The figure shows three views and two pictorial views of one solid part (mm, origin at its lowest corner). Answer the questions. A direction names the side the tool comes from. Coordinates: 2 decimals unless noted, no trailing zeros. Loops run counter-clockwise (first coordinate to the right, second up) from the corner with the lowest first, then second, coordinate; pieces in that order, holes last. Notation, with made-up numbers: M 29.25,52 L 86.25,52 A26 cw 86.25,75 Z; hole C 84.25,27 d6. An arc over 180 degrees is marked long. Answer as a JSON object with one key per item and string values. Group by question number.
1. For the marked faces 5, 6 and 7, determine the directions among +Z, -Z, +X, -X, +Y, -Y from which every point of the face is accessible in a straight line to the end or side of a thin tool.
2. Determine the mould class of the marked faces 1, 2, 3 and 4 for opening direction Z: released by +Z, released by -Z, zero draft, split by the parting line, or undercut.
3. A cutting plane is placed at A-A on x = 70. Give the vertices of the cut face in (y, z), and give its area (3 significant figures).
4. Straight lines are drawn through the part: L1, parallel to X at y = 8, z = 30; L2, parallel to X at y = 11.5, z = 38.5; L3, parallel to Z at x = 108, y = 5. For each, find the intervals that lie inside material, in ascending order.
5. Given pin 1 (6 mm diameter, centred on x = 29, y = 12, fed in from +Z); pin 2 (10 mm diameter, centred on y = 6, z = 24, fed in from +X); pin 3 (4 mm diameter, centred on y = 4, z = 34.5, fed in from -X); pin 4 (8 mm diameter, centred on x = 103, z = 52.5, fed in from -Y), each flat-ended and moving along its own axis, determine where each tip first touches the part or whether it passes through.
6. A cutting plane is placed at B-B on y = 11. Give the vertices of the cut face in (x, z), and give its area (3 significant figures).
7. A cutting plane is placed at C-C on z = 30. Give the vertices of the cut face in (x, y).
8. A cutting plane is placed at D-D on x = 35.5. Give the vertices of the cut face in (y, z).
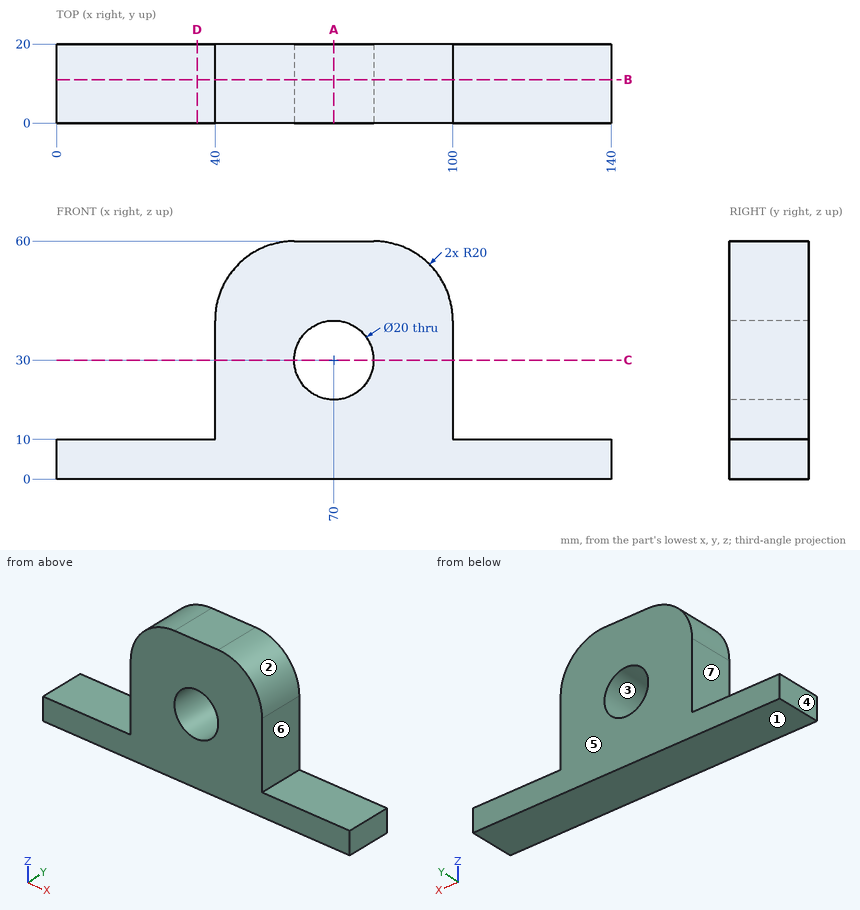
From the geometry:
{
 "1": {"face 5": "+Z, -Z, +X, -X, +Y", "face 6": "+Z, +X, +Y, -Y", "face 7": "+Z, -X, +Y, -Y"},
 "2": {"face 1": "released by -Z", "face 2": "released by +Z", "face 3": "undercut", "face 4": "zero draft"},
 "3": {"outline": "M 0,0 L 20,0 L 20,20 L 0,20 Z; M 0,40 L 20,40 L 20,60 L 0,60 Z", "area": "800 mm²"},
 "4": {"L1": "x = 40 to 60, 80 to 100", "L2": "x = 40 to 64.73, 75.27 to 100", "L3": "z = 0 to 10"},
 "5": {"pin 1": "stops at z = 10", "pin 2": "stops at x = 100", "pin 3": "stops at x = 40", "pin 4": "passes through"},
 "6": {"outline": "M 0,0 L 140,0 L 140,10 L 100,10 L 100,40 A20 ccw 80,60 L 60,60 A20 ccw 40,40 L 40,10 L 0,10 Z; hole C 70,30 d20", "area": "3,910 mm²"},
 "7": {"outline": "M 40,0 L 60,0 L 60,20 L 40,20 Z; M 80,0 L 100,0 L 100,20 L 80,20 Z"},
 "8": {"outline": "M 0,0 L 20,0 L 20,10 L 0,10 Z"}
}
